```python
from build123d import *

# Parameters (mm, degrees)
F0_R     = 31.75
F1_DEPTH = 609.6
F3_DEPTH = 304.8


with BuildPart() as f1:
    # F0 (on Top) → F1 (new body, symmetric)
    with BuildSketch(Plane.XY):
        Circle(F0_R)
    extrude(amount=F1_DEPTH, both=True)

    # F2 (on face) → F3 (cut)
    with BuildSketch(Plane.XY.offset(609.6)):
        with BuildLine():
            Line((29.099356, 12.7), (-29.099356, 12.7))
            ThreePointArc((-29.099356, 12.7), (-31.75, 0), (-29.099356, -12.7))
            Line((-29.099356, -12.7), (29.099356, -12.7))
            ThreePointArc((29.099356, -12.7), (31.75, 0), (29.099356, 12.7))
        make_face()
    extrude(amount=-F3_DEPTH, mode=Mode.SUBTRACT)


solid = f1.part
```
Geometry check sheet. Reference: the model listing, model coordinates, mm. A direction names the side the tool comes from. Give positions to 0.01 mm unless a question says otherwise; leave off trailing zeros. Order: outer loops, then holes, each group sorted by start corner. A loop starts at its lowest first (then second) coordinate and runs counter-clockwise, first axis right, second up.
1. Section check C-C, the plane y = 0. Enter the section's corners in (x, z), and give its area (3 significant figures).
2. Release check for a two-part mould opening along Y. For faces 1 (the face through (0, 12.7, 459)), 2 (the face through (0, 20, 609.6)), 3 (the face through (-31.72, 1.4, 8.53)) record: pulls with the +Y half, pulls with the -Y half, needs draft (parallel to the pull), parting line crosses it, or undercut.
3. Section check B-B, the plane z = 391. Enter the section's corners in (x, y), and give its area (3 significant figures).
4. Thickness scan on L1, parallel to Y at x = -2.5, z = 442.5; L2, parallel to Y at x = -9, z = 517.5; L3, parallel to Z at x = 4.5, y = -12.5. Record the ranges inside material, lowest first.
5. Access from +Z, -Z, +X, -X, +Y, -Y to the whole of each face (thin tool, end or side, straight path). Record for faces 4 (the face through (0, 0, -609.6)), 5 (the face through (0, 0, 304.8)).
6. Section check D-D, the plane z = -452.5. Enter the section's corners in (x, y).
7. Gauge pin test, flat ends, axial feed: pin 1 Ø4 at (x, z) = (-18.5, 259.5) entering from +Y; pin 2 Ø10 at (y, z) = (10.5, -431.5) entering from +X; pin 3 Ø12 at (x, z) = (20.5, -99) entering from -Y. Record the tip position at first contact, or that the pin passes through.
8. Section check A-A, the plane x = 0. Enter the section's corners in (y, z), and give its area (3 significant figures).
Values follow:
1. outline: (-31.75, -609.6) - (31.75, -609.6) - (31.75, 304.8) - (-31.75, 304.8) - close
1. area: 58,100 mm2
2. face 1: undercut
2. face 2: needs draft
2. face 3: parting line crosses it
3. outline: (-29.1, -12.7) arc R31.75 ccw to (29.1, -12.7) - close; (-29.1, 12.7) - (29.1, 12.7) arc R31.75 ccw to start
3. area: 1,600 mm2
4. L1: y = -31.65 to -12.7, 12.7 to 31.65
4. L2: y = -30.45 to -12.7, 12.7 to 30.45
4. L3: z = -609.6 to 304.8
5. face 4: -Z, +X, -X, +Y, -Y
5. face 5: +Z, +X, -X
6. outline: circle Ø63.5 at (0, 0)
7. pin 1: stops at y = 27.13
7. pin 2: stops at x = 31.27
7. pin 3: stops at y = -28.25
8. outline: (-31.75, -609.6) - (31.75, -609.6) - (31.75, 609.6) - (12.7, 609.6) - (12.7, 304.8) - (-12.7, 304.8) - (-12.7, 609.6) - (-31.75, 609.6) - close
8. area: 69,700 mm2
